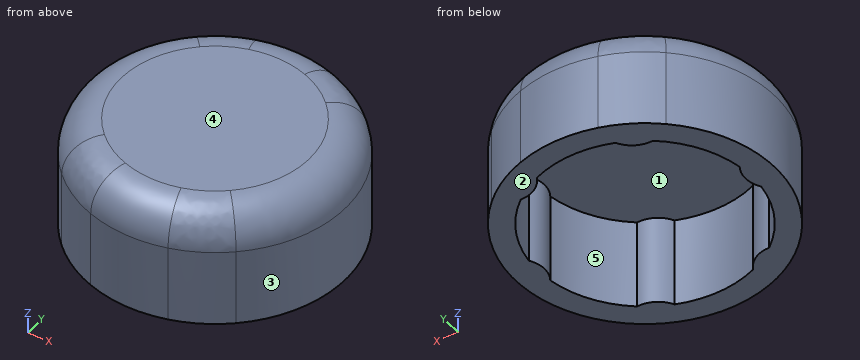
from build123d import *

# Parameters (mm, degrees)
F1_R     = 18.2626
F1_R_2   = 15.0876
F2_DEPTH = 12.7
F3_R     = 18.2626
F4_DEPTH = 3.175
F6_DEPTH = 12.7
F7_R     = 5.08


with BuildPart() as f2:
    # F1 (on Top) → F2 (new body)
    with BuildSketch(Plane.XY):
        Circle(F1_R)
        Circle(F1_R_2, mode=Mode.SUBTRACT)
    extrude(amount=F2_DEPTH)

    # F3 (on face) → F4 (join)
    with BuildSketch(Plane.XY.offset(12.7)):
        Circle(F3_R)
    extrude(amount=F4_DEPTH)

    # F5 (on face) → F6 (join, through all)
    with BuildSketch(Plane(origin=(0, 0, 0), x_dir=(1, 0, 0), z_dir=(0, 0, -1))):
        with BuildLine():
            ThreePointArc((-17.827214, 3.963961), (-18.2626, 0), (-17.827214, -3.963961))
            ThreePointArc((-17.827214, -3.963961), (-14.2748, 0), (-17.827214, 3.963961))
        make_face()
        with BuildLine():
            ThreePointArc((-12.346498, -13.45684), (-9.1313, -15.815876), (-5.480716, -17.420801))
            ThreePointArc((-5.480716, -17.420801), (-7.1374, -12.362339), (-12.346498, -13.45684))
        make_face()
        with BuildLine():
            ThreePointArc((5.480716, -17.420801), (9.1313, -15.815876), (12.346498, -13.45684))
            ThreePointArc((12.346498, -13.45684), (7.1374, -12.362339), (5.480716, -17.420801))
        make_face()
        with BuildLine():
            ThreePointArc((17.827214, -3.963961), (18.2626, 0), (17.827214, 3.963961))
            ThreePointArc((17.827214, 3.963961), (14.2748, 0), (17.827214, -3.963961))
        make_face()
        with BuildLine():
            ThreePointArc((12.346498, 13.45684), (9.1313, 15.815876), (5.480716, 17.420801))
            ThreePointArc((5.480716, 17.420801), (7.1374, 12.362339), (12.346498, 13.45684))
        make_face()
        with BuildLine():
            ThreePointArc((-5.480716, 17.420801), (-9.1313, 15.815876), (-12.346498, 13.45684))
            ThreePointArc((-12.346498, 13.45684), (-7.1374, 12.362339), (-5.480716, 17.420801))
        make_face()
    extrude(amount=-F6_DEPTH)

    # F7
    f7_edges = [f2.edges().sort_by_distance(p)[0] for p in [
        (-18.2626, 0, 15.875),
    ]]
    fillet(f7_edges, radius=F7_R)


solid = f2.part
Input: part model. Units: mm. Frame: model coordinates. Face numbers are marked on the shaded views. A direction names the side the tool comes from. Give positions to 0.01 mm unless a question says otherwise; leave off trailing zeros. Loops run counter-clockwise (first coordinate to the right, second up) from the corner with the lowest first, then second, coordinate; pieces in that order, holes last. Notation, with made-up numbers: (35, 28) -> (53, 28) arc R19 cw to (53, 46) -> close; hole circle Ø6 at (-15.75, 3). An arc over 180 degrees is marked (long way). Answer as a JSON object with one key per item and string values. Group by question number.
Item 1: Line query: probe 1 along Z at (x, y) = (-12.5, 3) (3 decimals); probe 2 along X at (y, z) = (-4, 8.5); probe 3 along Y at (x, z) = (6.5, 8.75). Output: solid intervals per line, ascending.
Item 2: Pin query (flat end, axial travel): P1, Ø2, axis at y = 13.5, z = 2, coming from the -X side; P2, Ø5, axis at y = 5.5, z = 13.5, coming from the +X side; P3, Ø1.5, axis at x = 11, z = 10.5, coming from the +Y side; P4, Ø2, axis at x = -14.5, y = 9.5, coming from the -Z side. Return the tip coordinate at first contact, or that it passes through.
Item 3: Reachability of the marked faces 1 and 2 from +Z, -Z, +X, -X, +Y, -Y: full face, straight path, thin tool, end or side. Return the list, or none.
Item 4: Pull-direction query (X, two-part tool) for the marked faces 3, 4 and 5; classes: released by +X, released by -X, zero draft, split by the parting line, or undercut.
Item 5: Cut plane A-A, the plane z = 9. Return the cut outline in (x, y).
Checks:
{
 "1": {"probe 1": "z = 12.7 to 15.875", "probe 2": "x = -17.82 to -14.55, 14.55 to 17.82", "probe 3": "y = -17.07 to -12.82, 12.82 to 17.07"},
 "2": {"P1": "stops at x = -13.31", "P2": "stops at x = 17.79", "P3": "stops at y = 15.11", "P4": "stops at z = 0"},
 "3": {"face 1": "-Z", "face 2": "-Z, +X, -X, +Y, -Y"},
 "4": {"face 3": "released by +X", "face 4": "zero draft", "face 5": "undercut"},
 "5": {"outline": "(-12.35, -13.46) arc R18.26 ccw to (-5.48, -17.42) arc R18.26 ccw to (5.48, -17.42) arc R18.26 ccw to (12.35, -13.46) arc R18.26 ccw to (12.35, 13.46) arc R18.26 ccw to (5.48, 17.42) arc R18.26 ccw to (-5.48, 17.42) arc R18.26 ccw to (-12.35, 13.46) arc R18.26 ccw to start; hole (-14.93, -2.19) arc R15.09 ccw to (-9.36, -11.83) arc R3.99 cw to (-5.57, -14.02) arc R15.09 ccw to (5.57, -14.02) arc R3.99 cw to (9.36, -11.83) arc R15.09 ccw to (14.93, -2.19) arc R3.99 cw to (14.93, 2.19) arc R15.09 ccw to (9.36, 11.83) arc R3.99 cw to (5.57, 14.02) arc R15.09 ccw to (-5.57, 14.02) arc R3.99 cw to (-9.36, 11.83) arc R15.09 ccw to (-14.93, 2.19) arc R3.99 cw to start"}
}
